```python
from build123d import *

# Parameters (mm, degrees)
CROQUIS1_R              = 1.499999985
CROQUIS1_R_2            = 1.499999871
SALIENTE_EXTRUIR1_DEPTH = 4


with BuildPart() as part:
    # Croquis1 → Saliente-Extruir1 (new body)
    with BuildSketch(Plane(origin=(0, 0, 0), x_dir=(1, 0, 0), z_dir=(0, 1, 0))):
        with BuildLine():
            Line((-12.499997978, -1.290428922), (-12.499997978, -3.618590638))
            Line((-12.499997978, -3.618590638), (12.500000954, -3.618590638))
            Line((12.500000954, -3.618590638), (12.500000954, -1.290428922))
            Line((12.500000954, -1.290428922), (8.627905846, 1.868327334))
            ThreePointArc((8.627905846, 1.868327334), (7.259690403, 2.621201307), (5.71991749, 2.881839161))
            Line((5.71991749, 2.881839161), (-5.687424356, 2.937856323))
            ThreePointArc((-5.687424356, 2.937856323), (-7.251897096, 2.662171308), (-8.627901793, 1.868327334))
            Line((-8.627901793, 1.868327334), (-12.499997978, -1.290428922))
        make_face()
        with Locations((-5.449998151, -0.648590639)):
            Circle(CROQUIS1_R, mode=Mode.SUBTRACT)
        with Locations((5.750001083, -0.64859061)):
            Circle(CROQUIS1_R_2, mode=Mode.SUBTRACT)
    extrude(amount=SALIENTE_EXTRUIR1_DEPTH)


solid = part.part
```
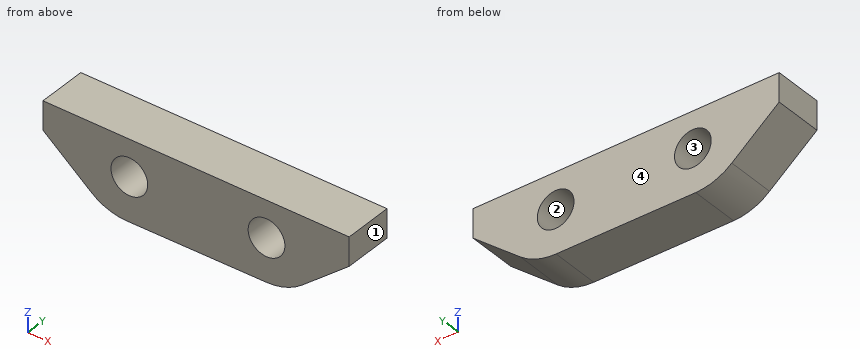
Design review of the part built by this model. Coordinates are the model's own, in mm. Face numbers are marked on the shaded views. Coordinates: 2 decimals unless noted, no trailing zeros. Order: outer loops, then holes, each group sorted by start corner. A loop starts at its lowest first (then second) coordinate and runs counter-clockwise, first axis right, second up.
1) Take a section at D-D, the plane x = 10.25. Give the boundary of the cut face in (y, z), and give its area (3 significant figures).
2) Take a section at C-C, the plane y = 3.55. Give the boundary of the cut face in (x, z).
3) Mouldability with a two-part tool opening along X and no side actions: class the marked faces 1, 2, 3 and 4 as +X half, -X half, draft (parallel to the pull), parting line (faces both ways), or undercut.
4) Wall thickness on line 1 along X through (y, z) = (0.35, 0); line 2 along X through (y, z) = (1.15, 0.5); line 3 along Z through (x, y) = (-6.5, 2.35): over which ranges is each line inside the solid? List them lowest first.
5) Take a section at B-B, the plane x = 6.75. Give the boundary of the cut face in (y, z), and give its area (3 significant figures).
6) Take a section at A-A, the plane z = 1. Give the boundary of the cut face in (x, y), and give its area (3 significant figures).
Returned:
1. outline: (0, -0.55) - (4, -0.55) - (4, 3.62) - (0, 3.62) - close
1. area: 16.7 mm2
2. outline: (-12.5, 1.29) - (-8.63, -1.87) arc R4.58 ccw to (-5.69, -2.94) - (5.72, -2.88) arc R4.68 ccw to (8.63, -1.87) - (12.5, 1.29) - (12.5, 3.62) - (-12.5, 3.62) - close; hole circle Ø3 at (-5.45, 0.65); hole circle Ø3 at (5.75, 0.65)
3. face 1: +X half
3. face 2: undercut
3. face 3: undercut
3. face 4: draft
4. line 1: x = -10.92 to -6.8, -4.1 to 4.4, 7.1 to 10.92
4. line 2: x = -11.53 to -6.94, -3.96 to 4.26, 7.24 to 11.53
4. line 3: z = -2.87 to -0.42, 1.72 to 3.62
5. outline: (0, -2.77) - (4, -2.77) - (4, -0.47) - (0, -0.47) - close; (0, 1.77) - (4, 1.77) - (4, 3.62) - (0, 3.62) - close
5. area: 16.6 mm2
6. outline: (-12.14, 0) - (-6.91, 0) - (-6.91, 4) - (-12.14, 4) - close; (-3.99, 0) - (4.29, 0) - (4.29, 4) - (-3.99, 4) - close; (7.21, 0) - (12.14, 0) - (12.14, 4) - (7.21, 4) - close
6. area: 73.8 mm2
